from build123d import *

# Parameters (mm, degrees)
PCB_W               = 18.5
PCB_H               = 15
PCB_R               = 1
BOSS_EXTRUDE1_DEPTH = 1


with BuildPart() as part:
    # PCB → Boss-Extrude1 (new body)
    with BuildSketch(Plane.XY):
        Rectangle(PCB_W, PCB_H)
        with Locations((-4.25, 5.5)):
            Circle(PCB_R, mode=Mode.SUBTRACT)
        with Locations((-4.25, -5.5)):
            Circle(PCB_R, mode=Mode.SUBTRACT)
    extrude(amount=BOSS_EXTRUDE1_DEPTH)


solid = part.part
For this review, take the finished solid that the model builds, in its own axes (mm). Round coordinates to 2 decimals unless told otherwise and drop trailing zeros. Loops run counter-clockwise (first coordinate to the right, second up) from the corner with the lowest first, then second, coordinate; pieces in that order, holes last. Notation, with made-up numbers: (-27.5, 38) - (-1.5, 38) arc R12 ccw to (-1.5, 52) - close; hole circle Ø1 at (67.5, 15). An arc over 180 degrees is marked (long way). Put each result on its own line as item: value. Start each with the question number.
1. Consider section C-C on z = 0.85. State the section outline as (x, y) points.
2. Consider section A-A on y = -5.5. State the section outline as (x, z) points, plus the area to 3 significant figures.
3. For probe 1 along Y at (x, z) = (-4.25, 0.6); probe 2 along Y at (x, z) = (-5, 0.1), list the stretches that pass through material, from the lowest coordinate up. Write a range as [from, to].
4. Mouldability with a two-part tool opening along X and no side actions: class faces 1 (the flat face through (0, 0, 1)), 2 (the flat face through (-9.25, -0.1, 0.5)), 3 (the cylindrical face through (-4.38, 6.49, 0.49)) as +X half, -X half, draft (parallel to the pull), parting line (faces both ways), or undercut.
5. Consider section B-B on x = -4.25. State the section outline as (y, z) points.
Result sheet:
1. outline: (-9.25, -7.5) - (9.25, -7.5) - (9.25, 7.5) - (-9.25, 7.5) - close; hole circle Ø2 at (-4.25, -5.5); hole circle Ø2 at (-4.25, 5.5)
2. outline: (-9.25, 0) - (-5.25, 0) - (-5.25, 1) - (-9.25, 1) - close; (-3.25, 0) - (9.25, 0) - (9.25, 1) - (-3.25, 1) - close
2. area: 16.5 mm^2
3. probe 1: [-7.5, -6.5], [-4.5, 4.5], [6.5, 7.5]
3. probe 2: [-7.5, -6.16], [-4.84, 4.84], [6.16, 7.5]
4. face 1: draft
4. face 2: -X half
4. face 3: undercut
5. outline: (-7.5, 0) - (-6.5, 0) - (-6.5, 1) - (-7.5, 1) - close; (-4.5, 0) - (4.5, 0) - (4.5, 1) - (-4.5, 1) - close; (6.5, 0) - (7.5, 0) - (7.5, 1) - (6.5, 1) - close
